Study the drawing (mm; zero at the part's minimum x, y, z) and answer. Give positions to 0.01 mm unless a question says otherwise; leave off trailing zeros. Write each loop counter-clockwise with the first axis right and the second up, starting at its lowest first coordinate (ties: lowest second). Pieces come first, ordered by that corner, then holes. Notation, with made-up numbers: (13.5, 37.5) - (19.5, 37.5) arc R19 ccw to (19.5, 66.5) - close; hole circle Ø11 at (56, -26.5). An arc over 180 degrees is marked (long way). Return JSON: item names as keys, results as strings.
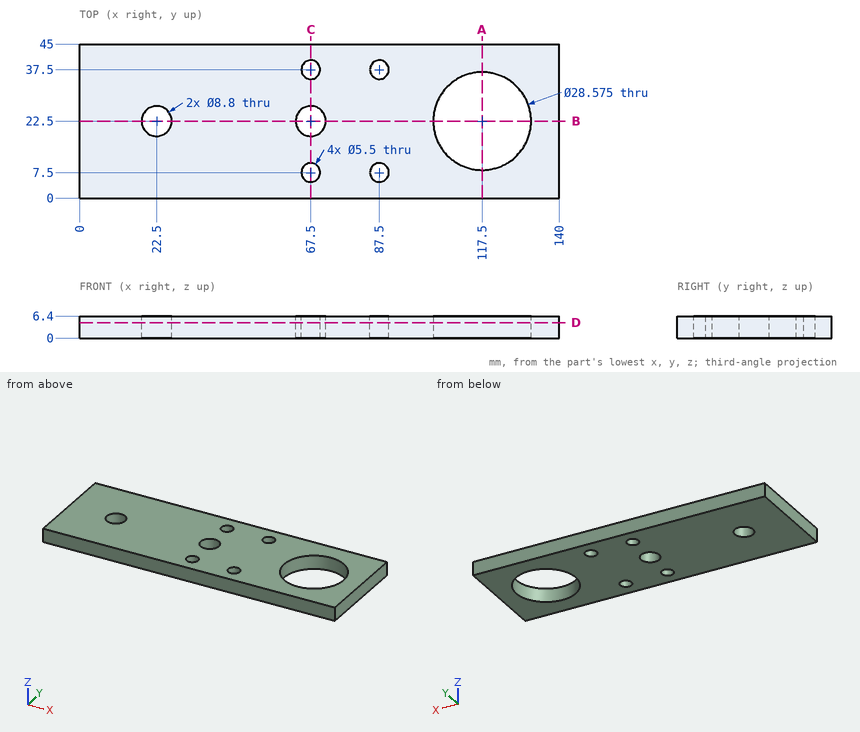
Item 1: A cutting plane is placed at B-B on y = 22.5. Determine the outline of the cut face in (x, z).
Answer below:
{"outline": "(0, 0) - (18.1, 0) - (18.1, 6.4) - (0, 6.4) - close; (26.9, 0) - (63.1, 0) - (63.1, 6.4) - (26.9, 6.4) - close; (71.9, 0) - (103.21, 0) - (103.21, 6.4) - (71.9, 6.4) - close; (131.79, 0) - (140, 0) - (140, 6.4) - (131.79, 6.4) - close"}
Item 2: A cutting plane is placed at A-A on x = 117.5. Determine the outline of the cut face in (y, z), then the cut area to 3 significant figures.
Answer below:
{"outline": "(0, 0) - (8.21, 0) - (8.21, 6.4) - (0, 6.4) - close; (36.79, 0) - (45, 0) - (45, 6.4) - (36.79, 6.4) - close", "area": "105 mm²"}
Item 3: A cutting plane is placed at C-C on x = 67.5. Determine the outline of the cut face in (y, z), then the cut area to 3 significant figures.
Answer below:
{"outline": "(0, 0) - (4.75, 0) - (4.75, 6.4) - (0, 6.4) - close; (10.25, 0) - (18.1, 0) - (18.1, 6.4) - (10.25, 6.4) - close; (26.9, 0) - (34.75, 0) - (34.75, 6.4) - (26.9, 6.4) - close; (40.25, 0) - (45, 0) - (45, 6.4) - (40.25, 6.4) - close", "area": "161 mm²"}
Item 4: A cutting plane is placed at D-D on z = 4.5. Give the number of separate pieces and of enclosed holes in the cut face, then the cut area to 3 significant figures.
Answer below:
{"separate pieces": "1", "enclosed holes": "7", "area": "5,440 mm²"}
Item 5: Consider L1, parallel to Y at x = 67.5, z = 2.5; L2, parallel to X at y = 23.5, z = 5; L3, parallel to X at y = 7.5, z = 3. Determine where each line is inside the solid, lowest interval first.
Answer below:
{"L1": "y = 0 to 4.75, 10.25 to 18.1, 26.9 to 34.75, 40.25 to 45", "L2": "x = 0 to 18.22, 26.78 to 63.22, 71.78 to 103.25, 131.75 to 140", "L3": "x = 0 to 64.75, 70.25 to 84.75, 90.25 to 140"}
